```python
from build123d import *

# Parameters (mm, degrees)
SKETCH2_R           = 5.5
SKETCH2_R_2         = 2.5
BOSS_EXTRUDE1_DEPTH = 2
SKETCH4_R           = 5
SKETCH4_R_2         = 3.5
CUT_EXTRUDE1_DEPTH  = 0.5


with BuildPart() as part:
    # Sketch2 → Boss-Extrude1 (new body)
    with BuildSketch(Plane.XY):
        with Locations((5.726371269, 6.63304672)):
            Circle(SKETCH2_R)
        with Locations((5.726371269, 6.63304672)):
            Circle(SKETCH2_R_2, mode=Mode.SUBTRACT)
    boss_extrude1 = extrude(amount=BOSS_EXTRUDE1_DEPTH)

    # Sketch4 → Cut-Extrude1 (cut)
    with BuildSketch(Plane.XY.offset(2)):
        with Locations((5.726371269, 6.63304672)):
            Circle(SKETCH4_R)
        with Locations((5.726371269, 6.63304672)):
            Circle(SKETCH4_R_2, mode=Mode.SUBTRACT)
    cut_extrude1 = extrude(amount=-CUT_EXTRUDE1_DEPTH, mode=Mode.SUBTRACT)

    # Mirror2: Boss-Extrude1, Cut-Extrude1 across plane
    add(boss_extrude1.mirror(Plane(origin=(5.726371269, 6.63304672, 0), x_dir=(1, 0, 0), z_dir=(0, 0, 1))))
    add(cut_extrude1.mirror(Plane(origin=(5.726371269, 6.63304672, 0), x_dir=(1, 0, 0), z_dir=(0, 0, 1))), mode=Mode.SUBTRACT)


solid = part.part
```
Geometry check sheet. Reference: the model listing, model coordinates, mm. A direction names the side the tool comes from. Coordinates: 2 decimals unless noted, no trailing zeros. Order: outer loops, then holes, each group sorted by start corner. A loop starts at its lowest first (then second) coordinate and runs counter-clockwise, first axis right, second up.
Q1. Draft check along Y on faces 4 (the face through (4.642, 1.752, -1.754)), 5 (the face through (5.01, 12.086, 0.028)), 6 (the face through (3, 7, 2)). Enter one of: released by +Y, released by -Y, zero draft, split by the parting line, or undercut.
Reply:
face 4: undercut
face 5: split by the parting line
face 6: zero draft
Q2. Thickness scan on probe 1 along X at (y, z) = (6.75, -1.8) (3 decimals); probe 2 along X at (y, z) = (6.5, -0.8); probe 3 along Y at (x, z) = (7, 1.8). Record the ranges inside material, lowest first.
Reply:
probe 1: x = 0.228 to 0.728, 2.228 to 3.229, 8.224 to 9.224, 10.725 to 11.225
probe 2: x = 0.23 to 3.23, 8.22 to 11.22
probe 3: y = 1.28 to 1.8, 3.37 to 4.48, 8.78 to 9.89, 11.47 to 11.98
Q3. Sectioned sample at B-B on y = 6.25. Record the cut outline in (x, z), and give its area (3 significant figures).
Reply:
outline: (0.24, -2) - (0.74, -2) - (0.74, -1.5) - (2.25, -1.5) - (2.25, -2) - (3.26, -2) - (3.26, 2) - (2.25, 2) - (2.25, 1.5) - (0.74, 1.5) - (0.74, 2) - (0.24, 2) - close; (8.2, -2) - (9.21, -2) - (9.21, -1.5) - (10.71, -1.5) - (10.71, -2) - (11.21, -2) - (11.21, 2) - (10.71, 2) - (10.71, 1.5) - (9.21, 1.5) - (9.21, 2) - (8.2, 2) - close
area: 21.1 mm2
Q4. Sectioned sample at C-C on y = 3. Record the cut outline in (x, z).
Reply:
outline: (1.6, -2) - (2.29, -2) - (2.29, -1.5) - (9.16, -1.5) - (9.16, -2) - (9.86, -2) - (9.86, 2) - (9.16, 2) - (9.16, 1.5) - (2.29, 1.5) - (2.29, 2) - (1.6, 2) - close
Q5. Tool access check on faces 1 (the face through (9.065, 7.684, -1.754)), 2 (the face through (3, 7, -2)), 3 (the face through (9.065, 7.684, 1.754)). Record the directions out of +Z, -Z, +X, -X, +Y, -Y that give a thin tool (end or side, any length) a straight path to the whole face; none if there is none.
Reply:
face 1: -Z
face 2: -Z, +X, -X, +Y, -Y
face 3: +Z
Q6. Sectioned sample at D-D on x = 8.5. Record the cut outline in (y, z).
Reply:
outline: (1.88, -2) - (2.47, -2) - (2.47, -1.5) - (4.5, -1.5) - (4.5, -2) - (8.77, -2) - (8.77, -1.5) - (10.79, -1.5) - (10.79, -2) - (11.38, -2) - (11.38, 2) - (10.79, 2) - (10.79, 1.5) - (8.77, 1.5) - (8.77, 2) - (4.5, 2) - (4.5, 1.5) - (2.47, 1.5) - (2.47, 2) - (1.88, 2) - close
Q7. Sectioned sample at A-A on x = 5.25. Record the cut outline in (y, z), and give its area (3 significant figures).
Reply:
outline: (1.15, -2) - (1.66, -2) - (1.66, -1.5) - (3.17, -1.5) - (3.17, -2) - (4.18, -2) - (4.18, 2) - (3.17, 2) - (3.17, 1.5) - (1.66, 1.5) - (1.66, 2) - (1.15, 2) - close; (9.09, -2) - (10.1, -2) - (10.1, -1.5) - (11.61, -1.5) - (11.61, -2) - (12.11, -2) - (12.11, 2) - (11.61, 2) - (11.61, 1.5) - (10.1, 1.5) - (10.1, 2) - (9.09, 2) - close
area: 21.2 mm2
